```python
from build123d import *

# Parameters (mm, degrees)
SKETCH1_W           = 66
SKETCH1_H           = 125.5
SKETCH1_R           = 5.75
SKETCH1_W_2         = 50.55
SKETCH1_H_2         = 25.705
SKETCH1_W_3         = 39.72
SKETCH1_H_3         = 53.61
SKETCH1_W_4         = 42.72
SKETCH1_H_4         = 56.61
SKETCH1_W_5         = 53.55
SKETCH1_H_5         = 28.705
BOSS_EXTRUDE1_DEPTH = 1.5
SKETCH1_3_W         = 42.72
SKETCH1_3_H         = 56.61
SKETCH1_3_W_2       = 39.72
SKETCH1_3_H_2       = 53.61
BOSS_EXTRUDE2_DEPTH = 0.000481454
SKETCH1_4_W         = 53.55
SKETCH1_4_H         = 28.705
SKETCH1_4_W_2       = 50.55
SKETCH1_4_H_2       = 25.705
BOSS_EXTRUDE3_DEPTH = 0.000481454
BOSS_EXTRUDE4_START = -27.234481
SKETCH1_5_W         = 69
SKETCH1_5_H         = 128.5
SKETCH1_5_W_2       = 66
SKETCH1_5_H_2       = 125.5
BOSS_EXTRUDE4_DEPTH = 28.734481
BOSS_EXTRUDE5_START = -27.234481
SKETCH1_6_W         = 69
SKETCH1_6_H         = 128.5
BOSS_EXTRUDE5_DEPTH = 1.5
SKETCH2_R           = 10
SKETCH2_W           = 5
SKETCH2_H           = 20
CUT_EXTRUDE1_DEPTH  = 1


with BuildPart() as part:
    # Sketch1 → Boss-Extrude1 (new body)
    # profile 1 of 3: a face of its own
    with BuildSketch(Plane.XY):
        with Locations((16.854577092, 44.967543122)):
            Rectangle(SKETCH1_W, SKETCH1_H)
        with Locations((38.500244774, 7.618926737)):
            Circle(SKETCH1_R, mode=Mode.SUBTRACT)
        with Locations((27.186536275, -3.694781762)):
            Circle(SKETCH1_R, mode=Mode.SUBTRACT)
        with Locations((16.854577092, 92.618043122)):
            Rectangle(SKETCH1_W_2, SKETCH1_H_2, mode=Mode.SUBTRACT)
        with Locations((16.854577092, 49.317142331)):
            Rectangle(SKETCH1_W_3, SKETCH1_H_3, mode=Mode.SUBTRACT)
        Polygon((4, -11), (-4, -11), (-4, -4), (-11, -4), (-11, 4), (-4, 4), (-4, 11), (4, 11), (4, 4), (11, 4), (11, -4), (4, -4), align=None, mode=Mode.SUBTRACT)
    # profile 2 of 3: a face of its own
    with BuildSketch(Plane.XY):
        with Locations((16.854577092, 49.317142331)):
            Rectangle(SKETCH1_W_4, SKETCH1_H_4)
        with Locations((16.854577092, 49.317142331)):
            Rectangle(SKETCH1_W_3, SKETCH1_H_3, mode=Mode.SUBTRACT)
    # profile 3 of 3: a face of its own
    with BuildSketch(Plane.XY):
        with Locations((16.854577092, 92.618043122)):
            Rectangle(SKETCH1_W_5, SKETCH1_H_5)
        with Locations((16.854577092, 92.618043122)):
            Rectangle(SKETCH1_W_2, SKETCH1_H_2, mode=Mode.SUBTRACT)
    extrude(amount=BOSS_EXTRUDE1_DEPTH)

    # Sketch1<3> → Boss-Extrude2 (add)
    with BuildSketch(Plane.XY):
        with Locations((16.854577092, 49.317142331)):
            Rectangle(SKETCH1_3_W, SKETCH1_3_H)
        with Locations((16.854577092, 49.317142331)):
            Rectangle(SKETCH1_3_W_2, SKETCH1_3_H_2, mode=Mode.SUBTRACT)
    extrude(amount=-BOSS_EXTRUDE2_DEPTH)

    # Sketch1<4> → Boss-Extrude3 (add)
    with BuildSketch(Plane.XY):
        with Locations((16.854577092, 92.618043122)):
            Rectangle(SKETCH1_4_W, SKETCH1_4_H)
        with Locations((16.854577092, 92.618043122)):
            Rectangle(SKETCH1_4_W_2, SKETCH1_4_H_2, mode=Mode.SUBTRACT)
    extrude(amount=-BOSS_EXTRUDE3_DEPTH)

    # Sketch1<5> → Boss-Extrude4 (add)
    with BuildSketch(Plane.XY.offset(BOSS_EXTRUDE4_START)):
        with Locations((16.854577092, 44.967543122)):
            Rectangle(SKETCH1_5_W, SKETCH1_5_H)
        with Locations((16.854577092, 44.967543122)):
            Rectangle(SKETCH1_5_W_2, SKETCH1_5_H_2, mode=Mode.SUBTRACT)
    extrude(amount=BOSS_EXTRUDE4_DEPTH)

    # Sketch1<6> → Boss-Extrude5 (add)
    with BuildSketch(Plane.XY.offset(BOSS_EXTRUDE5_START)):
        with Locations((16.854577092, 44.967543122)):
            Rectangle(SKETCH1_6_W, SKETCH1_6_H)
    extrude(amount=-BOSS_EXTRUDE5_DEPTH)

    # Sketch2 → Cut-Extrude1 (cut)
    with BuildSketch(Plane(origin=(0, 109.217543122, 0), x_dir=(1, 0, 0), z_dir=(0, 1, 0))):
        with Locations(Location((1.104577092, 14.434481454, 0), (0, 0, 270))):
            Circle(SKETCH2_R)
        with Locations((39.104577092, 14.434481454)):
            Rectangle(SKETCH2_W, SKETCH2_H)
    extrude(amount=-CUT_EXTRUDE1_DEPTH, mode=Mode.SUBTRACT)


solid = part.part
```
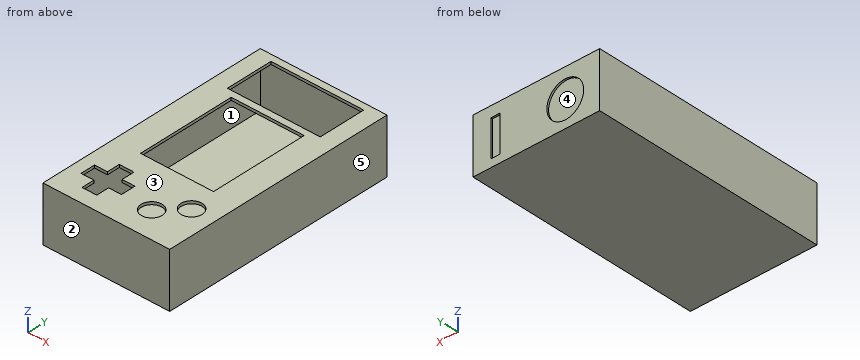
Geometry: final body of the model. Coordinates: model frame, mm. Face numbers are marked on the shaded views. A direction names the side the tool comes from. Round coordinates to 2 decimals unless told otherwise and drop trailing zeros. Write each loop counter-clockwise with the first axis right and the second up, starting at its lowest first coordinate (ties: lowest second). Pieces come first, ordered by that corner, then holes.
Item 1: Section query B-B (y = 16.5). Return loops of the section in (x, z).
Item 2: Material intervals for L1, parallel to X at y = 67, z = -26; L2, parallel to Y at x = 44, z = -4.5; L3, parallel to Z at x = 8.5, y = 7.5, sorted ascending.
Item 3: Pin query (flat end, axial travel): P1, Ø1, axis at x = 22.5, y = 84, coming from the +Z side. Return the tip coordinate at first contact, or that it passes through.
Item 4: Mould query, pull axis X, two halves, no side actions, for the marked faces 3, 4 and 5. Classes: +X half, -X half, draft (parallel to the pull), parting line (faces both ways), or undercut.
Item 5: Set-up query: the marked faces 1 and 2. Return all of +Z, -Z, +X, -X, +Y, -Y with unobstructed straight access to the full face (end or side cutting, diameter ignored); none if empty.
Item 6: Section query C-C (z = -26). Return loops of the section in (x, y).
Completed:
1. outline: (-17.65, -28.73) - (51.35, -28.73) - (51.35, 1.5) - (-17.65, 1.5) - close; hole (-16.15, -27.23) - (49.85, -27.23) - (49.85, 0) - (-16.15, 0) - close
2. L1: x = -17.65 to -16.15, 49.85 to 51.35
2. L2: y = -19.28 to -17.78, 107.72 to 109.22
2. L3: z = -28.73 to -27.23, 0 to 1.5
3. P1: stops at z = -27.23
4. face 3: draft
4. face 4: undercut
4. face 5: +X half
5. face 1: none
5. face 2: +Z, -Z, +X, -X, -Y
6. outline: (-17.65, -19.28) - (51.35, -19.28) - (51.35, 109.22) - (-17.65, 109.22) - close; hole (-16.15, -17.78) - (49.85, -17.78) - (49.85, 107.72) - (-16.15, 107.72) - close
